The listing builds one solid part. Answer for the finished solid, in the listing's coordinates (mm). Face numbers are marked on the shaded views. A direction names the side the tool comes from. Round coordinates to 2 decimals unless told otherwise and drop trailing zeros. Write each loop counter-clockwise with the first axis right and the second up, starting at its lowest first coordinate (ties: lowest second). Pieces come first, ordered by that corner, then holes. Notation, with made-up numbers: (-7.75, -7) - (18.25, -7) arc R10 ccw to (18.25, 11) - close; hole circle Ø8 at (51, 54.25). An arc over 180 degrees is marked (long way). Return JSON: item names as keys, results as strings. Group by question number.
from build123d import *

# Parameters (mm, degrees)
EXTRUDE_8_DEPTH     = 2
EXTRUDE_11_DEPTH    = 20
SKETCH_8_W          = 4
SKETCH_8_H          = 4
EXTRUDE_12_DEPTH    = 4
SKETCH_9_W          = 4
SKETCH_9_H          = 4
EXTRUDE_13_DEPTH    = 4
SKETCH_10_W         = 56
SKETCH_10_H         = 46
EXTRUDE_14_DEPTH    = 2.5
CUT_EXTRUDE_5_DEPTH = 60


with BuildPart() as part:
    # Эскиз1 → Бобышка-Вытянуть8 (new body)
    with BuildSketch(Plane.XY):
        with BuildLine():
            Line((-28, -25), (28, -25))
            ThreePointArc((28, -25), (29.414213562, -24.414213562), (30, -23))
            Line((30, -23), (30, 23))
            ThreePointArc((30, 23), (29.414213562, 24.414213562), (28, 25))
            Line((28, 25), (-28, 25))
            ThreePointArc((-28, 25), (-29.414213562, 24.414213562), (-30, 23))
            Line((-30, 23), (-30, -23))
            ThreePointArc((-30, -23), (-29.414213562, -24.414213562), (-28, -25))
        make_face()
    extrude(amount=EXTRUDE_8_DEPTH)

    # Эскиз6 → Бобышка-Вытянуть11 (add)
    with BuildSketch(Plane.XY.offset(2)):
        with BuildLine():
            Line((-28, 25), (28, 25))
            ThreePointArc((28, 25), (29.414213562, 24.414213562), (30, 23))
            Line((30, 23), (30, -23))
            ThreePointArc((30, -23), (29.414213562, -24.414213562), (28, -25))
            Line((28, -25), (-28, -25))
            ThreePointArc((-28, -25), (-29.414213562, -24.414213562), (-30, -23))
            Line((-30, -23), (-30, 23))
            ThreePointArc((-30, 23), (-29.414213562, 24.414213562), (-28, 25))
        make_face()
        Polygon((-28, -23), (28, -23), (28, 23), (-18, 23), (-18, 18), (-28, 18), align=None, mode=Mode.SUBTRACT)
    extrude(amount=EXTRUDE_11_DEPTH)

    # Эскиз8 → Бобышка-Вытянуть12 (add)
    with BuildSketch(Plane.XZ.offset(-23)):
        with Locations((26, 20)):
            Rectangle(SKETCH_8_W, SKETCH_8_H)
    extrude(amount=EXTRUDE_12_DEPTH)

    # Эскиз9 → Бобышка-Вытянуть13 (add)
    with BuildSketch(Plane(origin=(0, -23, 0), x_dir=(1, 0, 0), z_dir=(0, 1, 0))):
        with Locations((26, -20)):
            Rectangle(SKETCH_9_W, SKETCH_9_H)
        with Locations((-26, -20)):
            Rectangle(SKETCH_9_W, SKETCH_9_H)
    extrude(amount=EXTRUDE_13_DEPTH)

    # Эскиз10 → Бобышка-Вытянуть14 (add)
    with BuildSketch(Plane.XY.offset(22)):
        with BuildLine():
            Line((-28, 25), (28, 25))
            ThreePointArc((28, 25), (29.414213562, 24.414213562), (30, 23))
            Line((30, 23), (30, -23))
            ThreePointArc((30, -23), (29.414213562, -24.414213562), (28, -25))
            Line((28, -25), (-28, -25))
            ThreePointArc((-28, -25), (-29.414213562, -24.414213562), (-30, -23))
            Line((-30, -23), (-30, 23))
            ThreePointArc((-30, 23), (-29.414213562, 24.414213562), (-28, 25))
        make_face()
        Rectangle(SKETCH_10_W, SKETCH_10_H, mode=Mode.SUBTRACT)
    extrude(amount=EXTRUDE_14_DEPTH)

    # Эскиз15 → Вырез-Вытянуть5 (cut)
    with BuildSketch(Plane.ZY.offset(30)):
        with BuildLine():
            Line((8, 9), (8, -9))
            ThreePointArc((8, -9), (7, -10), (6, -9))
            Line((6, -9), (6, 9))
            ThreePointArc((6, 9), (7, 10), (8, 9))
        make_face()
        with BuildLine():
            Line((4, 9), (4, -9))
            ThreePointArc((4, -9), (3, -10), (2, -9))
            Line((2, -9), (2, 9))
            ThreePointArc((2, 9), (3, 10), (4, 9))
        make_face()
    extrude(amount=-CUT_EXTRUDE_5_DEPTH, mode=Mode.SUBTRACT)


solid = part.part
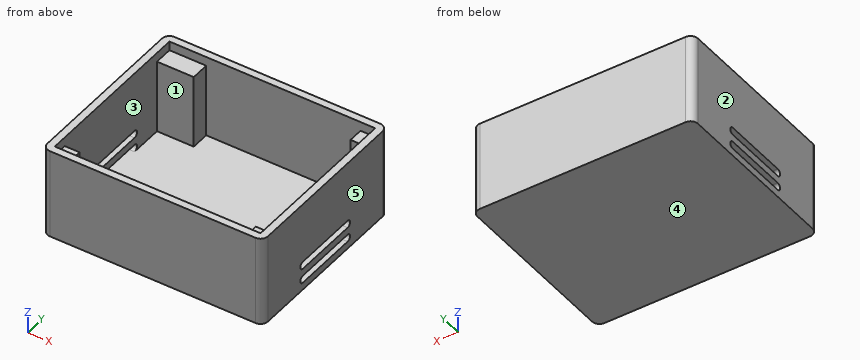
(1) Consider line 1 (Y direction, x = 27.5, z = 8); line 2 (X direction, y = -7.5, z = 21.25); line 3 (Y direction, x = -26, z = 12.5). Determine where each line is inside the solid, lowest interval first.
(2) Find section C-C (y = 13). Write down the section's boundary in (x, z).
(3) Flat-ended cylindrical pins translate along their axes: pin 1 (0.6 mm diameter, centred on x = 28.5, y = -2, fed in from -Z); pin 2 (6 mm diameter, centred on x = -4, y = 4.5, fed in from +Z); pin 3 (1.2 mm diameter, centred on x = -26, y = -21, fed in from +Z). Find the tip coordinate at first contact, or state that the pin passes through.
(4) For the marked faces 1 and 2, determine the directions among +Z, -Z, +X, -X, +Y, -Y from which every point of the face is accessible in a straight line to the end or side of a thin tool.
(5) Find section A-A (y = -2). Write down the section's boundary in (x, z), plus the area to 3 significant figures.
(6) Find section D-D (z = 10.5). Write down the section's boundary in (x, y).
(7) Find section B-B (z = 3). Write down the section's boundary in (x, y), plus the area to 3 significant figures.
(8) Determine the mould class of the marked faces 3, 4 and 5 for opening direction X: +X half, -X half, draft (parallel to the pull), parting line (faces both ways), or undercut.
Check sheet entries:
{
 "1": {"line 1": "y = -25 to -23, 23 to 25", "line 2": "x = -30 to -28, 28 to 30", "line 3": "y = -25 to -23, 18 to 25"},
 "2": {"outline": "(-30, 0) - (30, 0) - (30, 24.5) - (28, 24.5) - (28, 2) - (-28, 2) - (-28, 24.5) - (-30, 24.5) - close"},
 "3": {"pin 1": "stops at z = 0", "pin 2": "stops at z = 2", "pin 3": "stops at z = 22"},
 "4": {"face 1": "+Z", "face 2": "+Z, -Z, -X, +Y, -Y"},
 "5": {"outline": "(-30, 0) - (30, 0) - (30, 2) - (-30, 2) - close; (-30, 4) - (-28, 4) - (-28, 6) - (-30, 6) - close; (-30, 8) - (-28, 8) - (-28, 24.5) - (-30, 24.5) - close; (28, 4) - (30, 4) - (30, 6) - (28, 6) - close; (28, 8) - (30, 8) - (30, 24.5) - (28, 24.5) - close", "area": "194 mm^2"},
 "6": {"outline": "(-30, -23) arc R2 ccw to (-28, -25) - (28, -25) arc R2 ccw to (30, -23) - (30, 23) arc R2 ccw to (28, 25) - (-28, 25) arc R2 ccw to (-30, 23) - close; hole (-28, -23) - (28, -23) - (28, 23) - (-18, 23) - (-18, 18) - (-28, 18) - close"},
 "7": {"outline": "(-30, -23) arc R2 ccw to (-28, -25) - (28, -25) arc R2 ccw to (30, -23) - (30, -10) - (28, -10) - (28, -23) - (-28, -23) - (-28, -10) - (-30, -10) - close; (-30, 10) - (-28, 10) - (-28, 18) - (-18, 18) - (-18, 23) - (28, 23) - (28, 10) - (30, 10) - (30, 23) arc R2 ccw to (28, 25) - (-28, 25) arc R2 ccw to (-30, 23) - close", "area": "391 mm^2"},
 "8": {"face 3": "undercut", "face 4": "draft", "face 5": "+X half"}
}
